Source: CAD feature listing. Evaluate the final solid. Frame: model axes, mm. A direction names the side the tool comes from. Round coordinates to 2 decimals unless told otherwise and drop trailing zeros. Order: outer loops, then holes, each group sorted by start corner. A loop starts at its lowest first (then second) coordinate and runs counter-clockwise, first axis right, second up. Notation, with made-up numbers: (78.25, -28.75) -> (84.25, -28.75) arc R10 ccw to (84.25, -17.75) -> close; hole circle Ø6 at (67.25, 76.5). An arc over 180 degrees is marked (long way). Write item = value, one per line. Start each with the question number.
(1) Cut plane A-A on y = 10. Return the cut outline in (x, z).
(2) Cut plane D-D on y = 25. Return the cut outline in (x, z), then the cut area to 3 significant figures.
(3) Draft query along X for faces 4 (the face through (34.544, 10.826, 1.972)), 5 (the face through (41.921, 29, 2)), 6 (the face through (7, 9, 4)). Return one class per face: released by +X, released by -X, zero draft, split by the parting line, or undercut.
(4) Ray query, line 1 (Y direction, x = 35.5, z = 2.75); line 2 (X direction, y = -29, z = 3.15); line 3 (X direction, y = 54, z = 3.5). Return the intervals inside material, ascending.
(5) Cut plane C-C on x = 19. Return the cut outline in (y, z), then the cut area to 3 significant figures.
(6) Reachability of faces 1 (the face through (28, 0, 2)), 2 (the face through (-19.679, 8, 2)), 3 (the face through (32, 59.3, 2)) from +Z, -Z, +X, -X, +Y, -Y: full face, straight path, thin tool, end or side. Return the list, or none.
(7) Cut plane B-B on z = 1.8. Return the cut outline in (x, y), then the cut area to 3 significant figures.
(8) Contact query for flat-ended pins moving along their axis: pin 1 Ø1.2 at (y, z) = (53, 2) entering from -X; pin 2 Ø7 at (x, y) = (31.92, 10) entering from -Z. Output: stop coordinate, or through.
from build123d import *

# Parameters (mm, degrees)
SKETCH1_R           = 2.75
BOSS_EXTRUDE1_DEPTH = 4


with BuildPart() as part:
    # Sketch1 → Boss-Extrude1 (new body)
    with BuildSketch(Plane.XY):
        with BuildLine():
            Line((14.684243546, 0), (41.920581655, 0))
            Line((41.920581655, 0), (41.920581655, 59.3))
            Line((41.920581655, 59.3), (21.920581655, 59.3))
            Line((21.920581655, 59.3), (21.920581655, 39.3))
            Line((21.920581655, 39.3), (7.820581655, 39.3))
            ThreePointArc((7.820581655, 39.3), (-11.624854827, 31.245436483), (-19.679418345, 11.8))
            Line((-19.679418345, 11.8), (-19.679418345, 3.567882185))
            Line((-19.679418345, 3.567882185), (-27.059465895, -38.286447318))
            Line((-27.059465895, -38.286447318), (-7.363310835, -41.759410871))
            Line((-7.363310835, -41.759410871), (-2.549892132, -14.461156891))
            ThreePointArc((-2.549892132, -14.461156891), (3.435460376, -4.094222245), (14.684243546, 0))
        make_face()
        with Locations((31.920581655, 49.3)):
            Circle(SKETCH1_R, mode=Mode.SUBTRACT)
        with Locations((31.920581655, 25)):
            Circle(SKETCH1_R, mode=Mode.SUBTRACT)
        with Locations((31.920581655, 10)):
            Circle(SKETCH1_R, mode=Mode.SUBTRACT)
        with Locations((-15.474906589, -30.174851565)):
            Circle(SKETCH1_R, mode=Mode.SUBTRACT)
        with Locations((-12.870183924, -15.402735269)):
            Circle(SKETCH1_R, mode=Mode.SUBTRACT)
    extrude(amount=BOSS_EXTRUDE1_DEPTH)


solid = part.part
Evaluation:
q1.outline = (-19.68, 0) -> (29.17, 0) -> (29.17, 4) -> (-19.68, 4) -> close; (34.67, 0) -> (41.92, 0) -> (41.92, 4) -> (34.67, 4) -> close
q2.outline = (-16.3, 0) -> (29.17, 0) -> (29.17, 4) -> (-16.3, 4) -> close; (34.67, 0) -> (41.92, 0) -> (41.92, 4) -> (34.67, 4) -> close
q2.area = 211 mm^2
q3.face_4 = undercut
q3.face_5 = released by +X
q3.face_6 = zero draft
q4.line_1 = 0 to 59.3
q4.line_2 = -25.42 to -17.96, -12.99 to -5.11
q4.line_3 = 21.92 to 41.92
q5.outline = (0, 0) -> (39.3, 0) -> (39.3, 4) -> (0, 4) -> close
q5.area = 157 mm^2
q6.face_1 = +Z, -Z, +X, -Y
q6.face_2 = +Z, -Z, -X, +Y
q6.face_3 = +Z, -Z, +X, -X, +Y
q7.outline = (-27.06, -38.29) -> (-7.36, -41.76) -> (-2.55, -14.46) arc R17.5 cw to (14.68, 0) -> (41.92, 0) -> (41.92, 59.3) -> (21.92, 59.3) -> (21.92, 39.3) -> (7.82, 39.3) arc R27.5 ccw to (-19.68, 11.8) -> (-19.68, 3.57) -> close; hole circle Ø5.5 at (-15.47, -30.17); hole circle Ø5.5 at (-12.87, -15.4); hole circle Ø5.5 at (31.92, 10); hole circle Ø5.5 at (31.92, 25); hole circle Ø5.5 at (31.92, 49.3)
q7.area = 3,400 mm^2
q8.pin_1 = 21.92
q8.pin_2 = 0
